Can you work these out from the model? Positions are in its coordinate system, mm. A direction names the side the tool comes from. Coordinates: 2 decimals unless noted, no trailing zeros. Loops run counter-clockwise (first coordinate to the right, second up) from the corner with the lowest first, then second, coordinate; pieces in that order, holes last. Notation, with made-up numbers: (13.5, 54.5) -> (66.5, 54.5) arc R31 cw to (66.5, 88.5) -> close; hole circle Ø7 at (8, 82). An arc over 180 degrees is marked (long way). Use one line per item in the form item = value. Start each with the question number.
(1) Imagine slicing it at D-D (x = 14). List the corners of the cut face in (y, z) for me, plus the area to 3 significant figures.
(2) I'm going to push flat-ended pins straight in: pin 1 (1 mm diameter, centred on x = 6, z = 4.5, fed in from -Y); pin 2 (2 mm diameter, centred on y = 0, z = 8, fed in from +X); pin 3 (1.6 mm diameter, centred on x = 0.5, z = 8, fed in from +Y). Where does each tip first touch, or does it pass through?
(3) Imagine slicing it at A-A (y = 0). List the corners of the cut face in (x, z) for me, plus the area to 3 significant figures.
(4) On a 3-axis mill with a long thin cutter (end or side, diameter ignored), from which of +Z, -Z, +X, -X, +Y, -Y can I reach the whole of each face in a straight line? I mean faces 1 (the flat face through (0, 2.5, 7)), 2 (the flat face through (-2.5, 0, 7)), 3 (the flat face through (0, -2.5, 7)). Say none if no direction works.
(5) I need wall thicknesses on line 1 (Z direction, x = 2, y = -12); line 2 (Y direction, x = -0.5, z = 2.5); line 3 (Y direction, x = -14.5, z = 1.5). Which ranges of each line are inside material? Lowest first, please. Write a range as [from, to].
(6) Imagine slicing it at C-C (z = 3). List the corners of the cut face in (x, y) for me.
```python
from build123d import *

# Parameters (mm, degrees)
SKETCH1_R           = 17
BOSS_EXTRUDE1_DEPTH = 6.5
SKETCH2_W           = 5
SKETCH2_H           = 5
BOSS_EXTRUDE2_DEPTH = 2


with BuildPart() as part:
    # Sketch1 → Boss-Extrude1 (new body)
    with BuildSketch(Plane.XY):
        with Locations(Location((0, 0, 0), (0, 0, 180))):
            Circle(SKETCH1_R)
    extrude(amount=BOSS_EXTRUDE1_DEPTH)

    # Sketch2 → Boss-Extrude2 (add)
    with BuildSketch(Plane.XY.offset(6.5)):
        Rectangle(SKETCH2_W, SKETCH2_H)
    extrude(amount=BOSS_EXTRUDE2_DEPTH)


solid = part.part
```
Worked out:
q1.outline = (-9.64, 0) -> (9.64, 0) -> (9.64, 6.5) -> (-9.64, 6.5) -> close
q1.area = 125 mm2
q2.pin_1 = -16.09
q2.pin_2 = 2.5
q2.pin_3 = 2.5
q3.outline = (-17, 0) -> (17, 0) -> (17, 6.5) -> (2.5, 6.5) -> (2.5, 8.5) -> (-2.5, 8.5) -> (-2.5, 6.5) -> (-17, 6.5) -> close
q3.area = 231 mm2
q4.face_1 = +Z, +X, -X, +Y
q4.face_2 = +Z, -X, +Y, -Y
q4.face_3 = +Z, +X, -X, -Y
q5.line_1 = [0, 6.5]
q5.line_2 = [-16.99, 16.99]
q5.line_3 = [-8.87, 8.87]
q6.outline = circle Ø34 at (0, 0)
